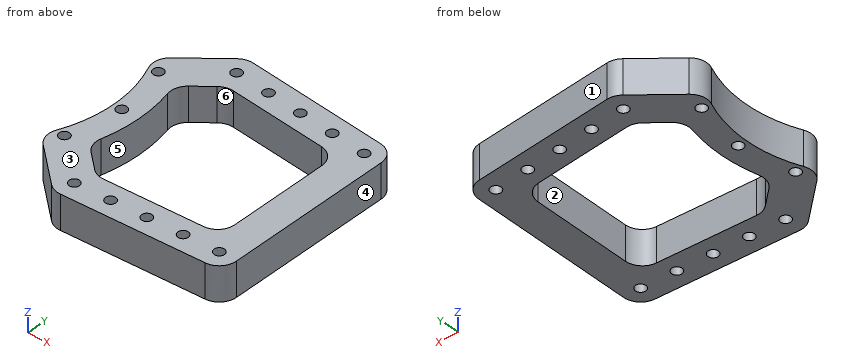
from build123d import *

# Parameters (mm, degrees)
EXTRUDE_1_DEPTH     = 15
FILLET_1_R          = 5
FILLET_2_R          = 5
FILLET_3_R          = 5
FILLET_4_R          = 5
FILLET_5_R          = 5
FILLET_6_R          = 5
FILLET_7_R          = 5
FILLET_8_R          = 5
FILLET_9_R          = 5
FILLET_10_R         = 5
FILLET_11_R         = 5
FILLET_12_R         = 5
FILLET_13_R         = 5
FILLET_14_R         = 5
FILLET_15_R         = 5
FILLET_16_R         = 5
SKETCH_5_R          = 1.5
CUT_EXTRUDE_1_DEPTH = 15
CUT_EXTRUDE_START   = -15
SKETCH_6_R          = 1.5
CUT_EXTRUDE_5_DEPTH = 15
EXTRUDE_2_DEPTH     = 15
FILLET_17_R         = 5
FILLET_18_R         = 5
FILLET_19_R         = 5
FILLET_20_R         = 5
SKETCH_8_W          = 96.520141499
SKETCH_8_H          = 72.316132992
CUT_EXTRUDE_6_DEPTH = 5


with BuildPart() as part:
    # 草图3 → 凸台-拉伸1 (new body)
    with BuildSketch(Plane.XY):
        with BuildLine():
            Line((101.99145665, -27.727634828), (114.18506552, -15.283623844))
            ThreePointArc((114.18506552, -15.283623844), (110, 0), (114.18506552, 15.283623844))
            Line((114.18506552, 15.283623844), (101.99145665, 27.727634828))
            Line((101.99145665, 27.727634828), (48.171786379, 31.57189699))
            Line((48.171786379, 31.57189699), (32.743622368, 18.278544642))
            ThreePointArc((32.743622368, 18.278544642), (37.5, 0), (32.743622368, -18.278544642))
            Line((32.743622368, -18.278544642), (48.171786379, -31.57189699))
            Line((48.171786379, -31.57189699), (101.99145665, -27.727634828))
        make_face()
        with BuildLine():
            ThreePointArc((42.839131819, -13.777110909), (45, 0), (42.839131819, 13.777110909))
            Line((42.839131819, 13.777110909), (51.574083604, 21.303398011))
            Line((51.574083604, 21.303398011), (97.500283316, 18.022955175))
            Line((97.500283316, 18.022955175), (106.212331228, 9.132000819))
            ThreePointArc((106.212331228, 9.132000819), (105, 0), (106.212331228, -9.132000819))
            Line((106.212331228, -9.132000819), (97.500283316, -18.022955175))
            Line((97.500283316, -18.022955175), (51.574083604, -21.303398011))
            Line((51.574083604, -21.303398011), (42.839131819, -13.777110909))
        make_face(mode=Mode.SUBTRACT)
    extrude(amount=EXTRUDE_1_DEPTH)

    # 圆角1
    fillet_1_edges = [part.edges().sort_by_distance(p)[0] for p in [
        (101.99145665, 27.727634828, 7.5),
    ]]
    fillet(fillet_1_edges, radius=FILLET_1_R)

    # 圆角2
    fillet_2_edges = [part.edges().sort_by_distance(p)[0] for p in [
        (114.18506552, 15.283623844, 7.5),
    ]]
    fillet(fillet_2_edges, radius=FILLET_2_R)

    # 圆角3
    fillet_3_edges = [part.edges().sort_by_distance(p)[0] for p in [
        (114.18506552, -15.283623844, 7.5),
    ]]
    fillet(fillet_3_edges, radius=FILLET_3_R)

    # 圆角4
    fillet_4_edges = [part.edges().sort_by_distance(p)[0] for p in [
        (101.99145665, -27.727634828, 7.5),
    ]]
    fillet(fillet_4_edges, radius=FILLET_4_R)

    # 圆角5
    fillet_5_edges = [part.edges().sort_by_distance(p)[0] for p in [
        (48.171786379, -31.57189699, 7.5),
    ]]
    fillet(fillet_5_edges, radius=FILLET_5_R)

    # 圆角6
    fillet_6_edges = [part.edges().sort_by_distance(p)[0] for p in [
        (48.171786379, 31.57189699, 7.5),
    ]]
    fillet(fillet_6_edges, radius=FILLET_6_R)

    # 圆角7
    fillet_7_edges = [part.edges().sort_by_distance(p)[0] for p in [
        (32.743622368, -18.278544642, 7.5),
    ]]
    fillet(fillet_7_edges, radius=FILLET_7_R)

    # 圆角8
    fillet_8_edges = [part.edges().sort_by_distance(p)[0] for p in [
        (32.743622368, 18.278544642, 7.5),
    ]]
    fillet(fillet_8_edges, radius=FILLET_8_R)

    # 圆角9
    fillet_9_edges = [part.edges().sort_by_distance(p)[0] for p in [
        (97.500283316, -18.022955175, 7.5),
    ]]
    fillet(fillet_9_edges, radius=FILLET_9_R)

    # 圆角10
    fillet_10_edges = [part.edges().sort_by_distance(p)[0] for p in [
        (106.212331228, -9.132000819, 7.5),
    ]]
    fillet(fillet_10_edges, radius=FILLET_10_R)

    # 圆角11
    fillet_11_edges = [part.edges().sort_by_distance(p)[0] for p in [
        (106.212331228, 9.132000819, 7.5),
    ]]
    fillet(fillet_11_edges, radius=FILLET_11_R)

    # 圆角12
    fillet_12_edges = [part.edges().sort_by_distance(p)[0] for p in [
        (97.500283316, 18.022955175, 7.5),
    ]]
    fillet(fillet_12_edges, radius=FILLET_12_R)

    # 圆角13
    fillet_13_edges = [part.edges().sort_by_distance(p)[0] for p in [
        (51.574083604, -21.303398011, 7.5),
    ]]
    fillet(fillet_13_edges, radius=FILLET_13_R)

    # 圆角14
    fillet_14_edges = [part.edges().sort_by_distance(p)[0] for p in [
        (42.839131819, -13.777110909, 7.5),
    ]]
    fillet(fillet_14_edges, radius=FILLET_14_R)

    # 圆角15
    fillet_15_edges = [part.edges().sort_by_distance(p)[0] for p in [
        (42.839131819, 13.777110909, 7.5),
    ]]
    fillet(fillet_15_edges, radius=FILLET_15_R)

    # 圆角16
    fillet_16_edges = [part.edges().sort_by_distance(p)[0] for p in [
        (51.574083604, 21.303398011, 7.5),
    ]]
    fillet(fillet_16_edges, radius=FILLET_16_R)

    # 草图5 → 切除-拉伸1 (cut)
    with BuildSketch(Plane(origin=(0, 0, 0), x_dir=(-1, 0, 0), z_dir=(0, 0, -1))):
        with Locations((-36.9551813, 15.307337295)):
            Circle(SKETCH_5_R)
        with Locations((-40, 0)):
            Circle(SKETCH_5_R)
        with Locations((-36.9551813, -15.307337295)):
            Circle(SKETCH_5_R)
        with Locations((-49.872934992, -26.437647501)):
            Circle(SKETCH_5_R)
        with Locations((-49.872934992, 26.437647501)):
            Circle(SKETCH_5_R)
        with Locations((-99.745869983, 22.875295001)):
            Circle(SKETCH_5_R)
        with Locations((-99.745869983, -22.875295001)):
            Circle(SKETCH_5_R)
        with Locations((-109.973915193, 12.437211552)):
            Circle(SKETCH_5_R)
        with Locations((-107.5, 0)):
            Circle(SKETCH_5_R)
        with Locations((-109.973915193, -12.437211552)):
            Circle(SKETCH_5_R)
        with Locations((-59.84752199, 25.725177001)):
            Circle(SKETCH_5_R)
        with Locations((-69.822108988, 25.012706501)):
            Circle(SKETCH_5_R)
        with Locations((-79.796695986, 24.300236001)):
            Circle(SKETCH_5_R)
        with Locations((-89.771282985, 23.587765501)):
            Circle(SKETCH_5_R)
        with Locations((-89.771282985, -23.587765501)):
            Circle(SKETCH_5_R)
        with Locations((-79.796695986, -24.300236001)):
            Circle(SKETCH_5_R)
        with Locations((-69.822108988, -25.012706501)):
            Circle(SKETCH_5_R)
        with Locations((-59.84752199, -25.725177001)):
            Circle(SKETCH_5_R)
    extrude(amount=-CUT_EXTRUDE_1_DEPTH, mode=Mode.SUBTRACT)

    # 草图6 → 切除-拉伸5 (cut)
    # profile 1 of 5: a face of its own
    with BuildSketch(Plane.XY.offset(15).offset(CUT_EXTRUDE_START)):
        with BuildLine():
            ThreePointArc((103.31715251, 26.374715112), (101.845820167, 27.412938577), (100.102105233, 27.8625885))
            Line((100.102105233, 27.8625885), (100.102105233, 24.332379915))
            ThreePointArc((100.102105233, 24.332379915), (100.925775249, 23.801482651), (101.245869983, 22.875295001))
            ThreePointArc((101.245869983, 22.875295001), (100.925775249, 21.949107351), (100.102105233, 21.418210087))
            Line((100.102105233, 21.418210087), (100.102105233, 15.367703489))
            Line((100.102105233, 15.367703489), (104.297377986, 11.086278624))
            ThreePointArc((104.297377986, 11.086278624), (105.514152308, 9.027175008), (105.635333526, 6.638501199))
            ThreePointArc((105.635333526, 6.638501199), (105, 0), (105.635333526, -6.638501199))
            ThreePointArc((105.635333526, -6.638501199), (105.514152308, -9.027175008), (104.297377986, -11.086278624))
            Line((104.297377986, -11.086278624), (100.102105233, -15.367703489))
            Line((100.102105233, -15.367703489), (100.102105233, -21.418210087))
            ThreePointArc((100.102105233, -21.418210087), (100.925775249, -21.949107351), (101.245869983, -22.875295001))
            ThreePointArc((101.245869983, -22.875295001), (100.925775249, -23.801482651), (100.102105233, -24.332379915))
            Line((100.102105233, -24.332379915), (100.102105233, -27.8625885))
            ThreePointArc((100.102105233, -27.8625885), (101.845820167, -27.412938577), (103.31715251, -26.374715112))
            Line((103.31715251, -26.374715112), (111.655402821, -17.865234485))
            ThreePointArc((111.655402821, -17.865234485), (113.00675492, -15.241981218), (112.643531681, -12.313555178))
            ThreePointArc((112.643531681, -12.313555178), (110, 0), (112.643531681, 12.313555178))
            ThreePointArc((112.643531681, 12.313555178), (113.00675492, 15.241981218), (111.655402821, 17.865234485))
            Line((111.655402821, 17.865234485), (103.31715251, 26.374715112))
        make_face()
        with Locations((109.973915193, -12.437211552)):
            Circle(SKETCH_6_R, mode=Mode.SUBTRACT)
        with Locations((107.5, 0)):
            Circle(SKETCH_6_R, mode=Mode.SUBTRACT)
        with Locations((109.973915193, 12.437211552)):
            Circle(SKETCH_6_R, mode=Mode.SUBTRACT)
    # profile 2 of 5: a face of its own
    with BuildSketch(Plane.XY.offset(15).offset(CUT_EXTRUDE_START)):
        with BuildLine():
            Line((100.102105233, -21.418210087), (100.102105233, -15.367703489))
            Line((100.102105233, -15.367703489), (98.825979176, -16.670035459))
            ThreePointArc((98.825979176, -16.670035459), (97.354646834, -17.708258924), (95.610931899, -18.157908847))
            Line((95.610931899, -18.157908847), (94.758576484, -18.218791377))
            Line((94.758576484, -18.218791377), (94.758576484, -23.231530251))
            Line((94.758576484, -23.231530251), (98.249681933, -22.982165576))
            ThreePointArc((98.249681933, -22.982165576), (98.778211836, -21.729154647), (100.102105233, -21.418210087))
        make_face()
    # profile 3 of 5: a face of its own
    with BuildSketch(Plane.XY.offset(15).offset(CUT_EXTRUDE_START)):
        with BuildLine():
            Line((94.758576484, -28.244269125), (100.102105233, -27.8625885))
            Line((100.102105233, -27.8625885), (100.102105233, -24.332379915))
            ThreePointArc((100.102105233, -24.332379915), (98.862330065, -24.087465457), (98.249681933, -22.982165576))
            Line((98.249681933, -22.982165576), (94.758576484, -23.231530251))
            Line((94.758576484, -23.231530251), (94.758576484, -28.244269125))
        make_face()
    # profile 4 of 5: a face of its own
    with BuildSketch(Plane.XY.offset(15).offset(CUT_EXTRUDE_START)):
        with BuildLine():
            Line((100.102105233, 15.367703489), (100.102105233, 21.418210087))
            ThreePointArc((100.102105233, 21.418210087), (98.778211836, 21.729154647), (98.249681933, 22.982165576))
            Line((98.249681933, 22.982165576), (94.758576484, 23.231530251))
            Line((94.758576484, 23.231530251), (94.758576484, 18.218791377))
            Line((94.758576484, 18.218791377), (95.610931899, 18.157908847))
            ThreePointArc((95.610931899, 18.157908847), (97.354646834, 17.708258924), (98.825979176, 16.670035459))
            Line((98.825979176, 16.670035459), (100.102105233, 15.367703489))
        make_face()
    # profile 5 of 5: a face of its own
    with BuildSketch(Plane.XY.offset(15).offset(CUT_EXTRUDE_START)):
        with BuildLine():
            Line((100.102105233, 24.332379915), (100.102105233, 27.8625885))
            Line((100.102105233, 27.8625885), (94.758576484, 28.244269125))
            Line((94.758576484, 28.244269125), (94.758576484, 23.231530251))
            Line((94.758576484, 23.231530251), (98.249681933, 22.982165576))
            ThreePointArc((98.249681933, 22.982165576), (98.862330065, 24.087465457), (100.102105233, 24.332379915))
        make_face()
    extrude(amount=CUT_EXTRUDE_5_DEPTH, mode=Mode.SUBTRACT)

    # 草图7 → 凸台-拉伸2 (add)
    with BuildSketch(Plane.XY.offset(15)):
        Polygon((94.758576484, -18.218791377), (94.758576484, 18.218791377), (85.826771952, 18.856777415), (85.826771952, -18.856777415), align=None)
    extrude(amount=-EXTRUDE_2_DEPTH)

    # 圆角17
    fillet_17_edges = [part.edges().sort_by_distance(p)[0] for p in [
        (94.758576484, 28.244269125, 7.5),
    ]]
    fillet(fillet_17_edges, radius=FILLET_17_R)

    # 圆角18
    fillet_18_edges = [part.edges().sort_by_distance(p)[0] for p in [
        (94.758576484, -28.244269125, 7.5),
    ]]
    fillet(fillet_18_edges, radius=FILLET_18_R)

    # 圆角19
    fillet_19_edges = [part.edges().sort_by_distance(p)[0] for p in [
        (85.826771952, 18.856777415, 7.5),
    ]]
    fillet(fillet_19_edges, radius=FILLET_19_R)

    # 圆角20
    fillet_20_edges = [part.edges().sort_by_distance(p)[0] for p in [
        (85.826771952, -18.856777415, 7.5),
    ]]
    fillet(fillet_20_edges, radius=FILLET_20_R)

    # 草图8 → 切除-拉伸6 (cut)
    with BuildSketch(Plane(origin=(0, 0, 0), x_dir=(-1, 0, 0), z_dir=(0, 0, -1))):
        with Locations((-67.250576804, -3.787424314)):
            Rectangle(SKETCH_8_W, SKETCH_8_H)
    extrude(amount=-CUT_EXTRUDE_6_DEPTH, mode=Mode.SUBTRACT)


solid = part.part
Geometry: final body of the model. Coordinates: model frame, mm. Face numbers are marked on the shaded views. A direction names the side the tool comes from. Coordinates: 2 decimals unless noted, no trailing zeros. Order: outer loops, then holes, each group sorted by start corner. A loop starts at its lowest first (then second) coordinate and runs counter-clockwise, first axis right, second up. Notation, with made-up numbers: (-14.5, 25) - (-7.5, 25) arc R21 ccw to (-7.5, 38) - close; hole circle Ø8 at (-25, 79). An arc over 180 degrees is marked (long way). Use one line per item in the form item = value.
1) Section B-B (x = 40). Return loops of the section in (y, z), then the cut area to 3 significant figures.
Solutions:
outline = (-24.53, 5) - (-1.5, 5) - (-1.5, 15) - (-24.53, 15) - close; (1.5, 5) - (24.53, 5) - (24.53, 15) - (1.5, 15) - close
area = 461 mm^2
2) Ray query, L1, parallel to X at y = -23, z = 14.75; L2, parallel to X at y = -14.5, z = 13; L3, parallel to Y at x = 60, z = 11.5. Return the intervals inside material, ascending.
Solutions:
L1 = 38.22 to 79.05, 80.54 to 88.39, 91.15 to 94.76
L2 = 34.58 to 35.69, 38.22 to 44.15, 85.82 to 94.76
L3 = -30.73 to -27.22, -24.23 to -20.7, 20.7 to 24.23, 27.22 to 30.73
3) Set-up query: the marked faces 1 and 2. Return all of +Z, -Z, +X, -X, +Y, -Y with unobstructed straight access to the full face (end or side cutting, diameter ignored); none if empty.
Solutions:
face_1 = +Z, -Z, +X, +Y
face_2 = +Z, -Z
4) Section D-D (z = 12.75). State how many separate pieces and enclosed holes the cut face has, then the cut area to 3 significant figures.
Solutions:
separate_pieces = 1
enclosed_holes = 14
area = 1,700 mm^2
5) Pin query (flat end, axial travel): pin 1 (2.5 mm diameter, centred on x = 89.77, y = -23.59, fed in from -Z); pin 2 (3 mm diameter, centred on y = 6, z = 11, fed in from -X); pin 3 (4 mm diameter, centred on x = 69.5, z = 7.5, fed in from +Y); pin 4 (3 mm diameter, centred on x = 79.5, z = 6.5, fed in from +Y). Return the tip coordinate at first contact, or that it passes through.
Solutions:
pin_1 = through
pin_2 = 36.74
pin_3 = 30.19
pin_4 = 29.44
6) Mould query, pull axis X, two halves, no side actions, for the marked faces 3, 4, 5 and 6. Classes: +X half, -X half, draft (parallel to the pull), parting line (faces both ways), or undercut.
Solutions:
face_3 = draft
face_4 = +X half
face_5 = undercut
face_6 = undercut
7) Section C-C (y = 7.5). Return loops of the section in (x, z), then the cut area to 3 significant figures.
Solutions:
outline = (36.74, 5) - (44.37, 5) - (44.37, 15) - (36.74, 15) - close; (85.83, 5) - (94.76, 5) - (94.76, 15) - (85.83, 15) - close
area = 166 mm^2
8) Section A-A (y = 0). Return loops of the section in (x, z), then the cut area to 3 significant figures.
Solutions:
outline = (37.5, 5) - (38.5, 5) - (38.5, 15) - (37.5, 15) - close; (41.5, 5) - (45, 5) - (45, 15) - (41.5, 15) - close; (85.83, 5) - (94.76, 5) - (94.76, 15) - (85.83, 15) - close
area = 134 mm^2
